```python
from build123d import *

# Parameters (mm, degrees)
F0_W      = 24
F0_H      = 14
F1_DEPTH  = 28
F2_W      = 4
F2_H      = 14
F3_DEPTH  = 14
F5_D      = 6
F6_R      = 6.99999
F7_R      = 5
F8_DEPTH  = 36
F9_R      = 2
F10_DEPTH = 100


# Not quite as in the source:
# - a fillet or chamfer is up to 0.001 mm smaller than in the source, because OpenCascade refuses the exact size


with BuildPart() as f1:
    # F0 (on Top) → F1 (new body)
    with BuildSketch(Plane.XY):
        with Locations((6.0259448364, -0.9606586885)):
            Rectangle(F0_W, F0_H)
    extrude(amount=-F1_DEPTH)

    # F2 (on face) → F3 (join)
    with BuildSketch(Plane.XY):
        with Locations((-3.9740551636, -0.9606586885)):
            Rectangle(F2_W, F2_H)
        with Locations((16.0259448364, -0.9606586885)):
            Rectangle(F2_W, F2_H)
    extrude(amount=F3_DEPTH)

    # F5 (through all)
    with Locations(Plane.YZ.offset(18.0259448364)):
        with Locations((-0.9606586885, 7)):
            Hole(F5_D / 2)

    # F6 (radius 7 in the source; OpenCascade refuses exactly that, so slightly less here)
    f6_edges = [f1.edges().sort_by_distance(p)[0] for p in [
        (16.025945, -7.960659, 14),
        (16.025945, 6.039341, 14),
        (-3.974055, 6.039341, 14),
        (-3.974055, -7.960659, 14),
    ]]
    fillet(f6_edges, radius=F6_R)

    # F7 (on face) → F8 (join)
    with BuildSketch(Plane(origin=(0, 0, -28), x_dir=(1, 0, 0), z_dir=(0, 0, -1))):
        with Locations((6.0259448364, 0.9606586885)):
            Circle(F7_R)
    extrude(amount=F8_DEPTH)

    # F9 (on face) → F10 (join)
    with BuildSketch(Plane(origin=(0, 0, -64), x_dir=(1, 0, 0), z_dir=(0, 0, -1))):
        with Locations((6.0259448364, 0.9606586885)):
            Circle(F9_R)
    extrude(amount=F10_DEPTH)


solid = f1.part
```
The model under review builds one solid part; all positions refer to its coordinate system, in mm. A direction names the side the tool comes from. Coordinates: 2 decimals unless noted, no trailing zeros. Write each loop counter-clockwise with the first axis right and the second up, starting at its lowest first coordinate (ties: lowest second). Pieces come first, ordered by that corner, then holes.
1) Machinability: for faces 1 (the face through (4.94, 3.92, -45.75)), 2 (the face through (6, -1, 0)), 3 (the face through (6, -1, -164)), which of the approach directions +Z, -Z, +X, -X, +Y, -Y give a long, thin tool a straight path to every point of the face, cutting with its end or side? Answer none if there is none.
2) We need section B-B on z = -139. State the section outline as (x, y) points, then the cut area to 3 significant figures.
3) We need section A-A on x = 12.5. State the section outline as (y, z) points.
4) To check wall thickness, follow probe 1 along Z at (x, y) = (10.25, -7); probe 2 along X at (y, z) = (-1, -88.5); probe 3 along Z at (x, y) = (4.75, -5.5). State the ranges of each line that lie inside material, in increasing order.
5) The part is to be moulded in two halves that separate along Y. For faces 4 (the face through (-4.002, 2.036, 7.132)), 5 (the face through (-3.95, -5.86, 12)), 6 (the face through (14.026, -1.1, 3.8)), say which applies: pulls with the +Y half, pulls with the -Y half, needs draft (parallel to the pull), parting line crosses it, or undercut.
6) Clearance check with flat-ended pins moving along their axes: pin 1 Ø8 at (x, y) = (4, -5.5) entering from +Z; pin 2 Ø4 at (x, z) = (11, -140) entering from -Y; pin 3 Ø1 at (x, y) = (9.5, 3) entering from -Z. State where each tip first meets the part, or that it passes through.
Answer list:
1. face 1: -Z
1. face 2: +Z, +Y, -Y
1. face 3: -Z, +X, -X, +Y, -Y
2. outline: circle Ø4 at (6.03, -0.96)
2. area: 12.6 mm2
3. outline: (-7.96, -28) - (6.04, -28) - (6.04, 0) - (-7.96, 0) - close
4. probe 1: z = -28 to 0
4. probe 2: x = 4.03 to 8.03
4. probe 3: z = -64 to 0
5. face 4: undercut
5. face 5: pulls with the -Y half
5. face 6: needs draft
6. pin 1: stops at z = 0
6. pin 2: passes through
6. pin 3: stops at z = -64
